Check sheet for the modelled part. Datum: model origin and axes. Units: mm. A direction names the side the tool comes from. Round coordinates to 2 decimals unless told otherwise and drop trailing zeros. Loops run counter-clockwise (first coordinate to the right, second up) from the corner with the lowest first, then second, coordinate; pieces in that order, holes last. Notation, with made-up numbers: M 13.5,89.5 L 65.5,89.5 A23 ccw 65.5,126.5 Z; hole C 21.25,5.25 d3. An arc over 180 degrees is marked long. Write item = value, one per line. Start each with the question number.
(1) Set-up check for faces 4 (the face through (27, 31, 0)), 5 (the face through (25.261, 34.304, 2.465)), 6 (the face through (0, 3, 1.5)), 7 (the face through (25.261, 33.973, -2.535)): record each of +Z, -Z, +X, -X, +Y, -Y from which the full face is reachable in a straight line by a thin tool's end or side.
(2) Cross-section at A-A on y = 39. Record the boundary of the cut face in (x, z), plus the area to 3 significant figures.
(3) Mould release check, pull along X, two halves, no side actions. Record for faces 1 (the face through (0, 40, 0)), 2 (the face through (0, 6, 0)), 3 (the face through (25, 22.32, 0)): pulls with the +X half, pulls with the -X half, needs draft (parallel to the pull), parting line crosses it, or undercut.
(4) Scan lines: L1, parallel to X at y = 27, z = 0; L2, parallel to X at y = 16, z = -13; L3, parallel to Z at x = -5, y = 29. Record each from-to range of solid material in increasing order. Write a range as from..to.
(5) Go/stop test with flat-tipped pins: P1, Ø2, axis at y = 11.5, z = 7.5, coming from the -X side; P2, Ø1, axis at y = 8.5, z = 12, coming from the +X side; P3, Ø12, axis at x = 1, z = -4, coming from the +Y side. Record where each tip stops, or that it passes through.
(6) Cross-section at C-C on z = -11. Record the boundary of the cut face in (x, y), plus the area to 3 significant figures.
(7) Cross-section at D-D on y = 32.5. Record the boundary of the cut face in (x, z), plus the area to 3 significant figures.
(8) Cross-section at B-B on x = -7. Record the boundary of the cut face in (y, z).
from build123d import *

# Parameters (mm, degrees)
SKETCH1_R                  = 24
SKETCH1_W                  = 5
SKETCH1_H                  = 3
BOSS_EXTRUDE1_DEPTH        = 6
BOSS_EXTRUDE4_OUTLINE_R    = 24
BOSS_EXTRUDE4_DEPTH        = 25.264714378
BOSS_EXTRUDE4_START        = 31.264714378
BOSS_EXTRUDE4_2_OUTLINE_R  = 24
BOSS_EXTRUDE4_2_DEPTH      = 17.470571244
BOSS_EXTRUDE4_START_2      = -55
BOSS_EXTRUDE4_3_OUTLINE_W  = 54
BOSS_EXTRUDE4_3_OUTLINE_H  = 50
BOSS_EXTRUDE4_3_DEPTH      = 17.412295169
BOSS_EXTRUDE5_REACH        = 64.39
BOSS_EXTRUDE5_START_RADIUS = 24
BOSS_EXTRUDE5_END_RADIUS   = 24


with BuildPart() as part:
    # Sketch1 → Boss-Extrude1 (new body)
    with BuildSketch(Plane(origin=(0, 0, 0), x_dir=(1, 0, 0), z_dir=(0, 1, 0))):
        with Locations(Location((0, 0, 0), (0, 0, 270))):
            Circle(SKETCH1_R)
        Rectangle(SKETCH1_W, SKETCH1_H, mode=Mode.SUBTRACT)
    extrude(amount=BOSS_EXTRUDE1_DEPTH)

    # Boss-Extrude4: read off the stored shape, not the designer's step
    # Boss-Extrude4 outline → Boss-Extrude4 (add)
    with BuildSketch(Plane(origin=(0, 6, 0), x_dir=(1, 0, 0), z_dir=(0, 1, 0))):
        Circle(BOSS_EXTRUDE4_OUTLINE_R)
    extrude(amount=BOSS_EXTRUDE4_DEPTH)

    # Boss-Extrude4 2 outline → Boss-Extrude4 2 (add)
    with BuildSketch(Plane(origin=(0, 0, 0), x_dir=(1, 0, 0), z_dir=(0, 1, 0)).offset(BOSS_EXTRUDE4_START)):
        Circle(BOSS_EXTRUDE4_2_OUTLINE_R)
    extrude(amount=BOSS_EXTRUDE4_2_DEPTH)

    # Boss-Extrude4 3 outline → Boss-Extrude4 3 (cut)
    with BuildSketch(Plane(origin=(0, 0, 0), x_dir=(0.9396926207859082, 0.3420201433256691, 0), z_dir=(0.3420201433256691, -0.9396926207859083, 0)).offset(BOSS_EXTRUDE4_START_2)):
        with Locations((14, 0)):
            Rectangle(BOSS_EXTRUDE4_3_OUTLINE_W, BOSS_EXTRUDE4_3_OUTLINE_H)
    extrude(amount=BOSS_EXTRUDE4_3_DEPTH, mode=Mode.SUBTRACT)

    # Boss-Extrude5: from a cylinder face, 64.39 long prism both ways, kept between that surface and its translate by the depth
    boss_extrude5_start = Plane(origin=(0, 30.19918, 0), z_dir=(0, -1, 0)) * Cylinder(BOSS_EXTRUDE5_START_RADIUS, 177.78, mode=Mode.PRIVATE)
    boss_extrude5_end = Plane(origin=(3, 30.19918, 0), z_dir=(0, -1, 0)) * Cylinder(BOSS_EXTRUDE5_END_RADIUS, 177.78, mode=Mode.PRIVATE)
    # Sketch5 → Boss-Extrude5 (add, from a surface)
    with BuildSketch(Plane(origin=(0, 0, 0), x_dir=(0, 0, -1), z_dir=(1, 0, 0)), mode=Mode.PRIVATE) as boss_extrude5_sk1:
        Polygon((0, 45.957345566), (-5, 22.320096474), (5, 22.320096474), align=None)
    boss_extrude5_tool1 = extrude(boss_extrude5_sk1.sketch, amount=BOSS_EXTRUDE5_REACH, both=True, mode=Mode.PRIVATE)
    add(((boss_extrude5_tool1 - boss_extrude5_start) & boss_extrude5_end).solids().sort_by_distance((25.236695, 30.19918, 0))[0])


solid = part.part
Result:
q1.face_4 = +X, +Y, -Y
q1.face_5 = +Z, +X, +Y
q1.face_6 = -Y
q1.face_7 = -Z, +X, +Y
q2.outline = M -2.75,-23.84 A24 ccw 23.95,-1.47 L 26.95,-1.47 A24 ccw 26.95,1.47 L 23.95,1.47 A24 ccw -2.75,23.84 Z
q2.area = 1,050 mm^2
q3.face_1 = pulls with the -X half
q3.face_2 = undercut
q3.face_3 = needs draft
q4.L1 = -24..27
q4.L2 = -20.17..20.17
q4.L3 = -23.47..23.47
q5.P1 = -23.1
q5.P2 = 21.07
q5.P3 = 42.55
q6.outline = M -21.33,0 L 21.33,0 L 21.33,47.76 L -21.33,32.24 Z
q6.area = 1,710 mm^2
q7.outline = M -20.61,-12.3 A24 ccw 23.83,-2.85 L 26.83,-2.85 A24 ccw 26.83,2.85 L 23.83,2.85 A24 ccw -20.61,12.3 Z
q7.area = 1,770 mm^2
q8.outline = M 0,-22.96 L 37.45,-22.96 L 37.45,22.96 L 0,22.96 Z
